Autodesk Inventor part; units mm, degrees
ref_plane "YZ Plane" through (0, 0, 0) normal (1, 0, 0) x (0, 1, 0)
ref_plane "XZ Plane" through (0, 0, 0) normal (0, 1, 0) x (-1, 0, 0)
ref_plane "XY Plane" through (0, 0, 0) normal (0, 0, 1) x (1, 0, 0)
sketch "Boceto31" plane through (0, 0, 0) normal (0, 1, 0) x (-1, 0, 0)
  line L0 (-58, 58) -> (58, 58)
  line L1 (58, 58) -> (58, -58)
  line L2 (58, -58) -> (-58, -58)
  line L3 (-58, -58) -> (-58, 58)
  line L4 (-58, 58) -> (58, -58) construction
  line L5 (58, 58) -> (-58, -58) construction
  line L6 (-32.5, 58) -> (32.5, 58)
  line L7 (32.5, 58) -> (32.5, -58)
  line L8 (32.5, -58) -> (-32.5, -58)
  line L9 (-32.5, -58) -> (-32.5, 58)
  line L10 (-32.5, 58) -> (32.5, -58) construction
  line L11 (32.5, 58) -> (-32.5, -58) construction
  line L12 (-48, 0) -> (48, 0) construction
  point P0 (0, 0)
  dimension "d155" = 116
  dimension "d156" = 116
  dimension "d157" = 65
  dimension "d158" = 96
extrude "Extrusión10" add sketch "Boceto31" against normal blind 10 contours L0 L9 L2 L3 | L0 L1 L2 L7
sketch "Boceto32" plane through (0, -10, 0) normal (0, -1, 0) x (1, 0, 0)
  line L0 (-32.5, 58) -> (-58, 58)
  line L1 (58, -58) -> (58, 58)
  line L2 (-58, 58) -> (58, 58)
  line L3 (58, 58) -> (58, -58)
  line L4 (58, -58) -> (-58, -58)
  line L5 (-58, -58) -> (-58, 58)
  point P0 (0, 0)
extrude "Extrusión11" add sketch "Boceto32" along normal blind 18 draft -30
hole "Agujero7" at (-48, 0, 0) at (48, 0, 0) direction (0, -1, 0) diameter 3.6 end through all
ref_plane "Plano de trabajo10" through (0, -18, 0) normal (0, -1, 0) x (1, 0, 0)
sketch "Boceto33" plane through (0, -18, 0) normal (0, -1, 0) x (1, 0, 0)
  line L0 (6.4663, 0) -> (3.2332, -5.6)
  line L1 (3.2332, -5.6) -> (-3.2332, -5.6)
  line L2 (-3.2332, -5.6) -> (-6.4663, 0)
  line L3 (-6.4663, 0) -> (-3.2332, 5.6)
  line L4 (-3.2332, 5.6) -> (3.2332, 5.6)
  line L5 (3.2332, 5.6) -> (6.4663, 0)
  point P0 (0, 0)
  point P1 (0, 0)
  dimension "d212" = 11.2
extrude "Extrusión12" cut sketch "Boceto33" along normal mid plane 12.8
sketch "Boceto34" plane through (0, -28, 0) normal (0, -1, 0) x (1, 0, 0)
  arc A0 (-47.6077, 1.7567) -> (-47.6077, -1.7567) centre (-48, 0) ccw
  circle A1 centre (-48, 0) radius 4
  line L0 (-17.8562, 0) -> (-10.0366, 0) construction
  circle A2 centre (48, 0) radius 4
  arc A3 (47.6077, -1.7567) -> (47.6077, 1.7567) centre (48, 0) ccw
  point P0 (0, 0)
  point P1 (0, 0)
  dimension "d194" = 8
  dimension "d197" = 96
hole "Agujero9" at (0, -28, 0) direction (0, 1, 0) diameter 9 depth 3.6
sketch "Boceto35" plane through (0, 0, 0) normal (0, 1, 0) x (1, 0, 0)
  line L0 (-58, -58) -> (-58, 58)
  line L1 (-58, 58) -> (-48, 58)
  line L2 (-48, 58) -> (-48, 48)
  line L3 (-48, 48) -> (-58, 48)
  line L4 (-58, 48) -> (-58, 58)
  line L5 (-32.5, 58) -> (-32.5, -58)
  line L6 (-32.5, 38) -> (-36.8198, 38)
  line L7 (-36.8198, 38) -> (-36.8198, 28)
  line L8 (-36.8198, 28) -> (-32.5, 28)
  line L9 (-32.5, 28) -> (-32.5, 38)
  line L10 (-32.5, 58) -> (-58, 58)
  point P0 (0, 0)
  dimension "d188" = 10
  dimension "d189" = 10
  dimension "d190" = 10
  dimension "d191" = 20
extrude "Extrusión13" cut sketch "Boceto35" against normal blind 3
mirror "Simetría2" about plane through (0, 0, 0) normal (1, 0, 0) of "Extrusión13"
mirror "Simetría3" about plane through (0, 0, 0) normal (0, 0, 1) of "Extrusión13", "Simetría2"
extrude "Extrusión14" cut sketch "Boceto34" against normal blind 20
sketch "Boceto37" plane through (0, -18, 0) normal (0, -1, 0) x (1, 0, 0)
  circle A0 centre (0, 0) radius 9.75
  dimension "d209" = 19.5
extrude "Extrusión16" cut sketch "Boceto37" along normal mid plane 1.64
properties part number "soporte_v2_3DPrint"
The model under review builds one solid part; all positions refer to its coordinate system, in mm. A direction names the side the tool comes from. Round coordinates to 2 decimals unless told otherwise and drop trailing zeros. Loops run counter-clockwise (first coordinate to the right, second up) from the corner with the lowest first, then second, coordinate; pieces in that order, holes last. Notation, with made-up numbers: (69.5, 68) - (112.5, 68) arc R31 cw to (112.5, 92) - close; hole circle Ø1 at (-32.5, 62.25). An arc over 180 degrees is marked (long way). Use a Markdown table: item, result. Add a question column.
Q1. The part is to be moulded in two halves that separate along Y. For faces 1 (the face through (4.827, -14.351, 2.839)), 2 (the face through (35, -3, -33)), 3 (the face through (44, -18, 0)), say which applies: pulls with the +Y half, pulls with the -Y half, needs draft (parallel to the pull), parting line crosses it, or undercut.
Q2. For probe 1 along X at (y, z) = (-1.75, 0); probe 2 along X at (y, z) = (-2, 45.5); probe 3 along X at (y, z) = (-1.75, 51.5), list the stretches that pass through material, from the lowest coordinate up.
Q3. Add section C-C (z = 18.5). State the section outline as (x, y) points.
Q4. Add section B-B (x = 0). State the section outline as (y, z) points, plus the area to 3 significant figures.
Q5. Machinability: for faces 4 (the face through (-48, -1, -53)), 5 (the face through (-36.82, -1, 33)), 6 (the face through (0, -22, 5.6)), 7 (the face through (0, -10, 1)), which of the approach directions +Z, -Z, +X, -X, +Y, -Y give a long, thin tool a straight path to every point of the face, cutting with its end or side? Answer none if there is none.
Q6. Insertion check: pin 1 Ø5 at (x, z) = (-54, -53) entering from +Y; pin 2 Ø3 at (x, z) = (0.5, 1) entering from -Y; pin 3 Ø8 at (y, z) = (-20, -21) entering from +X. Each pin has a flat end and moves straight along its axis. Give the tip position at first contact, or say it passes through.
Q7. Add section D-D (x = -17). State the section outline as (y, z) points.
Q8. Add section A-A (z = -33). State the section outline as (x, y) points, plus the area to 3 significant figures.
Worked answers:
| question | item | result |
|---|---|---|
| 1 | face 1 | undercut |
| 1 | face 2 | pulls with the +Y half |
| 1 | face 3 | needs draft |
| 2 | probe 1 | -58 to -49.8, -46.2 to -32.5, 32.5 to 46.2, 49.8 to 58 |
| 2 | probe 2 | -58 to -32.5, 32.5 to 58 |
| 2 | probe 3 | -48 to -32.5, 32.5 to 48 |
| 3 | outline | (-58, -10) - (-47.61, -28) - (47.61, -28) - (58, -10) - (58, 0) - (32.5, 0) - (32.5, -10) - (-32.5, -10) - (-32.5, 0) - (-58, 0) - close |
| 4 | outline | (-28, -47.61) - (-10, -58) - (-10, 58) - (-28, 47.61) - (-28, 4.5) - (-24.4, 4.5) - (-24.4, 5.6) - (-18.82, 5.6) - (-18.82, 9.75) - (-17.18, 9.75) - (-17.18, 5.6) - (-11.6, 5.6) - (-11.6, -5.6) - (-17.18, -5.6) - (-17.18, -9.75) - (-18.82, -9.75) - (-18.82, -5.6) - (-24.4, -5.6) - (-24.4, -4.5) - (-28, -4.5) - close |
| 4 | area | 1,710 mm² |
| 5 | face 4 | -Z, -X, +Y |
| 5 | face 5 | +Y |
| 5 | face 6 | none |
| 5 | face 7 | +Z, -Z, +Y |
| 6 | pin 1 | y = -3 |
| 6 | pin 2 | y = -11.6 |
| 6 | pin 3 | x = 54.54 |
| 7 | outline | (-28, -47.61) - (-10, -58) - (-10, 58) - (-28, 47.61) - close |
| 8 | outline | (-58, -10) - (-47.61, -28) - (47.61, -28) - (58, -10) - (58, 0) - (36.82, 0) - (36.82, -3) - (32.5, -3) - (32.5, -10) - (-32.5, -10) - (-32.5, -3) - (-36.82, -3) - (-36.82, 0) - (-58, 0) - close |
| 8 | area | 2,390 mm² |
